```python
from build123d import *

# Parameters (mm, degrees)
SKETCH1_W           = 304.8
SKETCH1_H           = 152.4
BOSS_EXTRUDE1_DEPTH = 0.79375
SKETCH2_R           = 2.25
CUT_EXTRUDE1_DEPTH  = 2.5875
SKETCH3_R           = 2.25
CUT_EXTRUDE2_DEPTH  = 2.5875
SKETCH4_R           = 1.7
CUT_EXTRUDE3_DEPTH  = 2.5875


with BuildPart() as part:
    # Sketch1 → Boss-Extrude1 (new body, symmetric)
    with BuildSketch(Plane.XY):
        Rectangle(SKETCH1_W, SKETCH1_H)
        Polygon((-120.65, 44.45), (-120.65, -44.45), (-31.75, 0), align=None, mode=Mode.SUBTRACT)
        Polygon((-78.052905029, 44.45), (78.052905029, 44.45), (0, 5.423547486), align=None, mode=Mode.SUBTRACT)
        Polygon((0, -5.423547486), (-78.052905029, -44.45), (78.052905029, -44.45), align=None, mode=Mode.SUBTRACT)
        Polygon((31.75, 0), (120.65, 44.45), (120.65, -44.45), align=None, mode=Mode.SUBTRACT)
    extrude(amount=BOSS_EXTRUDE1_DEPTH, both=True)

    # Sketch2 → Cut-Extrude1 (cut, through all)
    with BuildSketch(Plane.XY.offset(0.79375)):
        with Locations((133.355, 38.1)):
            Circle(SKETCH2_R)
        with Locations((133.355, 0)):
            Circle(SKETCH2_R)
        with Locations((133.355, -38.1)):
            Circle(SKETCH2_R)
        with Locations((114.3, 57.15)):
            Circle(SKETCH2_R)
        with Locations((114.3, -57.15)):
            Circle(SKETCH2_R)
        with Locations((76.2, -57.15)):
            Circle(SKETCH2_R)
        with Locations((76.2, 57.15)):
            Circle(SKETCH2_R)
        with Locations((38.1, -57.15)):
            Circle(SKETCH2_R)
        with Locations((38.1, 57.15)):
            Circle(SKETCH2_R)
        with Locations((0, -57.15)):
            Circle(SKETCH2_R)
        with Locations((0, 57.15)):
            Circle(SKETCH2_R)
        with Locations((-38.1, -57.15)):
            Circle(SKETCH2_R)
        with Locations((-38.1, 57.15)):
            Circle(SKETCH2_R)
        with Locations((-76.2, -57.15)):
            Circle(SKETCH2_R)
        with Locations((-76.2, 57.15)):
            Circle(SKETCH2_R)
        with Locations((-114.3, -57.15)):
            Circle(SKETCH2_R)
        with Locations((-114.3, 57.15)):
            Circle(SKETCH2_R)
        with Locations((130.175, 53.975)):
            Circle(SKETCH2_R)
        with Locations((138.641666667, 60.325)):
            Circle(SKETCH2_R)
        with Locations((130.175, -53.975)):
            Circle(SKETCH2_R)
        with Locations((138.641666667, -60.325)):
            Circle(SKETCH2_R)
    extrude(amount=-CUT_EXTRUDE1_DEPTH, mode=Mode.SUBTRACT)

    # Sketch3 → Cut-Extrude2 (cut, through all)
    with BuildSketch(Plane.XY.offset(0.79375)):
        with Locations((-146.05, 38.1)):
            Circle(SKETCH3_R)
        with Locations((-146.05, -38.1)):
            Circle(SKETCH3_R)
        with Locations((-146.05, 0)):
            Circle(SKETCH3_R)
    extrude(amount=-CUT_EXTRUDE2_DEPTH, mode=Mode.SUBTRACT)

    # Sketch4 → Cut-Extrude3 (cut, through all)
    with BuildSketch(Plane.XY.offset(0.79375)):
        with Locations((-101.6, -44.45)):
            Circle(SKETCH4_R)
        with Locations((101.6, -44.45)):
            Circle(SKETCH4_R)
        with Locations((101.6, 44.45)):
            Circle(SKETCH4_R)
        with Locations((-101.6, 44.45)):
            Circle(SKETCH4_R)
    extrude(amount=-CUT_EXTRUDE3_DEPTH, mode=Mode.SUBTRACT)


solid = part.part
```
Can you work these out from the model? Positions are in its coordinate system, mm. A direction names the side the tool comes from. Coordinates: 2 decimals unless noted, no trailing zeros. Loops run counter-clockwise (first coordinate to the right, second up) from the corner with the lowest first, then second, coordinate; pieces in that order, holes last. Notation, with made-up numbers: (26, 65) -> (63, 65) arc R25 cw to (63, 102) -> close; hole circle Ø4 at (-30, 44.5). An arc over 180 degrees is marked (long way). Put each result on its own line as item: value. Start each with the question number.
Q1. I want a section at C-C (x = 19). Write out the boundary of the cut face in (y, z), plus the area to 3 significant figures.
Q2. If I drill on line 1 (X direction, y = 11.5, z = -0.05); line 2 (Y direction, x = 38.1, z = 0.35) (3 decimals); line 3 (Y direction, x = -146.05, z = 0.3), over which ranges is the centre line in solid material (lowest first)? Write a range as [from, to].
Q3. I'm going to push flat-ended pins straight in: P1, Ø4, axis at x = -101.6, y = -44.45, coming from the -Z side; P2, Ø4, axis at x = -114.3, y = -57.15, coming from the -Z side. Where does each tip first touch, or does it pass through?
Q4. For faces 1 (the face through (-2, 1, 0.794)), 2 (the face through (76.822, -22.536, 0.011)), which set-ups out of +Z, -Z, +X, -X, +Y, -Y let a thin tool reach every point of the face, with its end or its side?
Q5. I want a section at A-A (x = 83). Write out the boundary of the cut face in (y, z) (3 decimals).
Q6. Thinking about a two-plate mould opening in Y: for faces 3 (the face through (75.578, 21.914, 0.011)), 4 (the face through (-2, 1, -0.794)), which applies, pulls with the +Y half, pulls with the -Y half, needs draft (parallel to the pull), parting line crosses it, or undercut?
Q7. I want a section at B-B (y = -11). Write out the boundary of the cut face in (x, z), plus the area to 3 significant figures.
Q8. I want a section at D-D (z = 0.1). Count the separate pieces of the cut face and the enclosed holes in it, plus the area to 3 significant figures.
Taken from the geometry:
1. outline: (-76.2, -0.79) -> (-44.45, -0.79) -> (-44.45, 0.79) -> (-76.2, 0.79) -> close; (-14.92, -0.79) -> (14.92, -0.79) -> (14.92, 0.79) -> (-14.92, 0.79) -> close; (44.45, -0.79) -> (76.2, -0.79) -> (76.2, 0.79) -> (44.45, 0.79) -> close
1. area: 148 mm2
2. line 1: x = [-152.4, -120.65], [-54.75, -12.15], [12.15, 54.75], [120.65, 152.4]
2. line 2: y = [-76.2, -59.4], [-54.9, -44.45], [-24.474, -3.175], [3.175, 24.474], [44.45, 54.9], [59.4, 76.2]
2. line 3: y = [-76.2, -40.35], [-35.85, -2.25], [2.25, 35.85], [40.35, 76.2]
3. P1: stops at z = -0.79
3. P2: passes through
4. face 1: +Z, +X, -X, +Y, -Y
4. face 2: +Z, -Z
5. outline: (-76.2, -0.794) -> (-25.625, -0.794) -> (-25.625, 0.794) -> (-76.2, 0.794) -> close; (25.625, -0.794) -> (76.2, -0.794) -> (76.2, 0.794) -> (25.625, 0.794) -> close
6. face 3: undercut
6. face 4: needs draft
7. outline: (-152.4, -0.79) -> (-120.65, -0.79) -> (-120.65, 0.79) -> (-152.4, 0.79) -> close; (-53.75, -0.79) -> (-11.15, -0.79) -> (-11.15, 0.79) -> (-53.75, 0.79) -> close; (11.15, -0.79) -> (53.75, -0.79) -> (53.75, 0.79) -> (11.15, 0.79) -> close; (120.65, -0.79) -> (152.4, -0.79) -> (152.4, 0.79) -> (120.65, 0.79) -> close
7. area: 236 mm2
8. separate pieces: 1
8. enclosed holes: 32
8. area: 32,000 mm2
